Here's how the part is built. I have some questions about the finished solid (model axes, mm). Coordinates: 2 decimals unless noted, no trailing zeros. Write each loop counter-clockwise with the first axis right and the second up, starting at its lowest first coordinate (ties: lowest second). Pieces come first, ordered by that corner, then holes. Notation, with made-up numbers: (72.5, 68) - (79.5, 68) arc R23 cw to (79.5, 96) - close; hole circle Ø10 at (-34, 56.5). An arc over 180 degrees is marked (long way). Answer in a Markdown table with one row per item. Add a question column.
Item 1: We'd pull the mould along Z, two halves only. Please class faces 1 (the face through (-14.82, 34.83, 9.59)), 2 (the face through (-53.56, 83.7, 5.14)), 3 (the face through (-16, 35, 9.2)), 4 (the face through (-49.7, 15.6, 0)): +Z half, -Z half, draft (parallel to the pull), parting line (faces both ways), or undercut.
Item 2: Imagine slicing it at C-C (x = -49). Please give me the cut outline in (y, z), plus the area to 3 significant figures.
Item 3: Imagine slicing it at A-A (y = 49). Please give me the cut outline in (x, z).
Item 4: I'm going to push flat-ended pins straight in: pin 1 (0.6 mm diameter, centred on x = -3.5, z = 0.5, fed in from +Y); pin 2 (12 mm diameter, centred on x = -18.5, y = 73.5, fed in from +Z); pin 3 (1.3 mm diameter, centred on y = 95.5, z = 0.5, fed in from -X); pin 4 (4 mm diameter, centred on x = -66, z = 3.5, fed in from +Y). Where does each tip first touch, or does it pass through?
Item 5: Imagine slicing it at B-B (x = -94.8). Please give me the cut outline in (y, z).
Item 6: If I drill on probe 1 along Y at (x, z) = (-94.8, 1.1); probe 2 along Y at (x, z) = (-49, 4); probe 3 along Z at (x, y) = (-5, 51.5), over which ranges is the centre line in solid material (lowest first)? Write a range as from..to.
Item 7: Imagine slicing it at D-D (z = 7.75). Please give me the cut outline in (x, y).
from build123d import *

# Parameters (mm, degrees)
BOSS_EXTRUDE1_DEPTH = 1.2
SKETCH2_R           = 1.65
CUT_EXTRUDE1_DEPTH  = 1.2
SKETCH3_R           = 35
BOSS_EXTRUDE2_DEPTH = 8
SKETCH5_R           = 37
BOSS_EXTRUDE3_DEPTH = 0.8
SKETCH6_R           = 32
CUT_EXTRUDE2_DEPTH  = 139.953229541
CHAMFER1_SIZE       = 1
CHAMFER2_SIZE       = 1


with BuildPart() as part:
    # Sketch1 → Boss-Extrude1 (new body)
    with BuildSketch(Plane(origin=(0, 0, 0), x_dir=(0, 1, 0), z_dir=(0, 0, 1))):
        Polygon((0, 8), (9, 8), (9, 0), (89, 0), (89, 8), (98, 8), (98, 90), (89, 90), (89, 98), (9, 98), (9, 90), (0, 90), align=None)
    extrude(amount=BOSS_EXTRUDE1_DEPTH)

    # Sketch2 → Cut-Extrude1 (cut)
    with BuildSketch(Plane.XY.offset(1.2)):
        with Locations((-94.8, 73.7)):
            Circle(SKETCH2_R)
        with Locations((-94.8, 24.3)):
            Circle(SKETCH2_R)
        with Locations((-3.2, 24.3)):
            Circle(SKETCH2_R)
        with Locations((-3.2, 73.7)):
            Circle(SKETCH2_R)
    extrude(amount=-CUT_EXTRUDE1_DEPTH, mode=Mode.SUBTRACT)

    # Sketch3 → Boss-Extrude2 (add)
    with BuildSketch(Plane.XY.offset(1.2)):
        with Locations((-49, 49)):
            Circle(SKETCH3_R)
    extrude(amount=BOSS_EXTRUDE2_DEPTH)

    # Sketch5 → Boss-Extrude3 (add)
    with BuildSketch(Plane.XY.offset(9.2)):
        with Locations((-49, 49)):
            Circle(SKETCH5_R)
    extrude(amount=BOSS_EXTRUDE3_DEPTH)

    # Sketch6 → Cut-Extrude2 (cut, through all)
    with BuildSketch(Plane.XY.offset(10)):
        with Locations((-49, 49)):
            Circle(SKETCH6_R)
    extrude(amount=-CUT_EXTRUDE2_DEPTH, mode=Mode.SUBTRACT)

    # Chamfer1
    chamfer1_edges = [part.edges().sort_by_distance(p)[0] for p in [
        (-4.85, 73.7, 0),
        (-4.85, 24.3, 0),
        (-96.45, 24.3, 0),
        (-96.45, 73.7, 0),
    ]]
    chamfer(chamfer1_edges, length=CHAMFER1_SIZE)

    # Chamfer2
    chamfer2_edges = [part.edges().sort_by_distance(p)[0] for p in [
        (-81, 49, 0),
        (-81, 49, 10),
    ]]
    chamfer(chamfer2_edges, length=CHAMFER2_SIZE)


solid = part.part
Here are the results:
| question | item | result |
|---|---|---|
| 1 | face 1 | draft |
| 1 | face 2 | undercut |
| 1 | face 3 | undercut |
| 1 | face 4 | -Z half |
| 2 | outline | (0, 0) - (16, 0) - (17, 1) - (17, 9) - (16, 10) - (12, 10) - (12, 9.2) - (14, 9.2) - (14, 1.2) - (0, 1.2) - close; (81, 1) - (82, 0) - (98, 0) - (98, 1.2) - (84, 1.2) - (84, 9.2) - (86, 9.2) - (86, 10) - (82, 10) - (81, 9) - close |
| 2 | area | 94.8 mm2 |
| 3 | outline | (-98, 0) - (-82, 0) - (-81, 1) - (-81, 9) - (-82, 10) - (-86, 10) - (-86, 9.2) - (-84, 9.2) - (-84, 1.2) - (-98, 1.2) - close; (-17, 1) - (-16, 0) - (0, 0) - (0, 1.2) - (-14, 1.2) - (-14, 9.2) - (-12, 9.2) - (-12, 10) - (-16, 10) - (-17, 9) - close |
| 4 | pin 1 | stops at y = 89 |
| 4 | pin 2 | stops at z = 10 |
| 4 | pin 3 | stops at x = -90 |
| 4 | pin 4 | stops at y = 80.62 |
| 5 | outline | (9, 0) - (21.65, 0) - (22.65, 1) - (22.65, 1.2) - (9, 1.2) - close; (25.95, 1) - (26.95, 0) - (71.05, 0) - (72.05, 1) - (72.05, 1.2) - (25.95, 1.2) - close; (75.35, 1) - (76.35, 0) - (89, 0) - (89, 1.2) - (75.35, 1.2) - close |
| 6 | probe 1 | y = 9..22.65, 25.95..72.05, 75.35..89 |
| 6 | probe 2 | y = 14..17, 81..84 |
| 6 | probe 3 | z = 0..1.2 |
| 7 | outline | circle Ø70 at (-49, 49); hole circle Ø64 at (-49, 49) |
